Job drawing, mm, ordinate dimensions from the low corner. One solid piece. A direction names the side the tool comes from. Coordinates: 2 decimals unless noted, no trailing zeros. Order: outer loops, then holes, each group sorted by start corner. A loop starts at its lowest first (then second) coordinate and runs counter-clockwise, first axis right, second up. Notation, with made-up numbers: M -16.5,-27 L -12.5,-27 A5 cw -12.5,-18 Z; hole C -37.5,62 d5. An arc over 180 degrees is marked long. Write item = value, one per line.
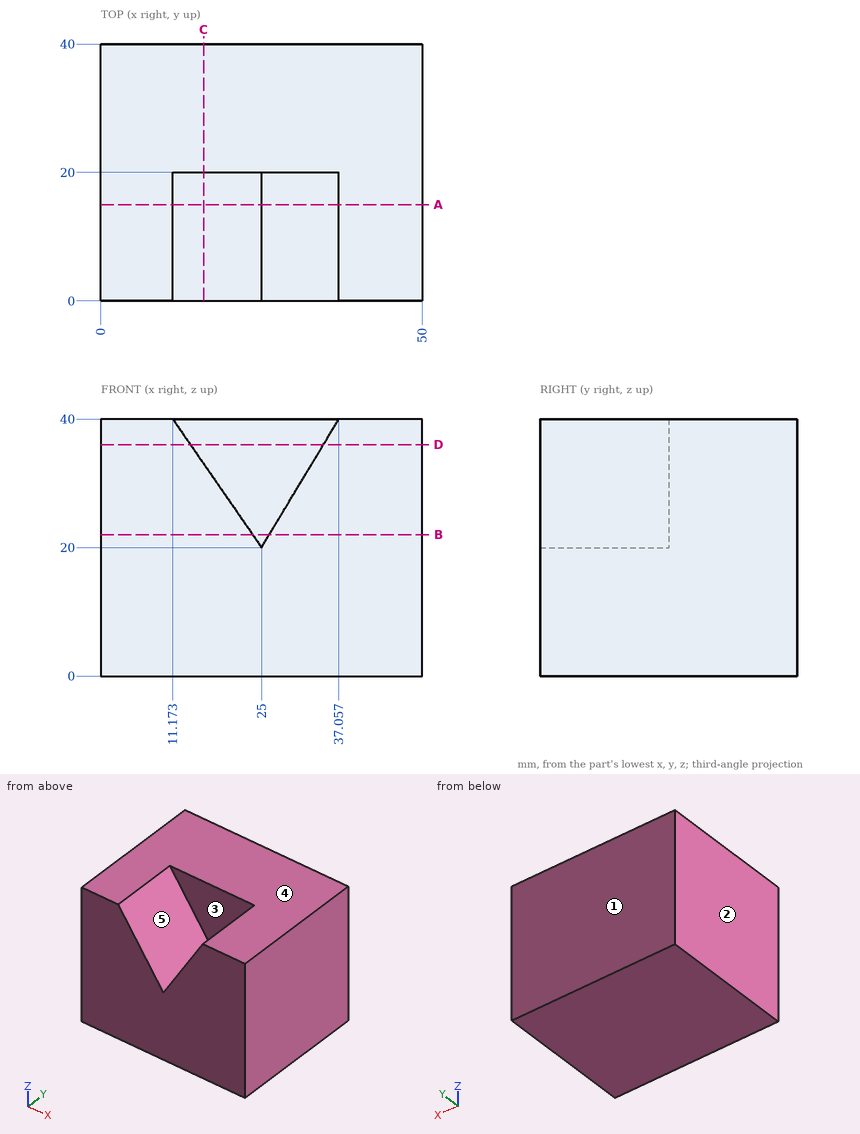
(1) Wall check: line 1 (Y direction, x = 27, z = 38.5); line 2 (X direction, y = 4, z = 26); line 3 (Z direction, x = 15, y = 13.5) (1 decimal). Give the ranges that are in metal, low to high. Write a range as from..to.
Evaluation:
line_1 = 20..40
line_2 = 0..20.85, 28.62..50
line_3 = 0..34.5
(2) Slice it at D-D, the plane z = 36. Write the cut outline in (x, y).
Evaluation:
outline = M 0,0 L 13.94,0 L 13.94,20 L 34.65,20 L 34.65,0 L 50,0 L 50,40 L 0,40 Z
(3) Tool access for the marked faces 4 and 5: list every direction of +Z, -Z, +X, -X, +Y, -Y with a clear straight run to the whole face (end or side of a thin tool).
Evaluation:
face_4 = +Z, +X, -X, +Y, -Y
face_5 = +Z, -Y
(4) Slice it at A-A, the plane y = 15. Write the cut outline in (x, z), then the cut area to 3 significant figures.
Evaluation:
outline = M 0,0 L 50,0 L 50,40 L 37.06,40 L 25,20 L 11.17,40 L 0,40 Z
area = 1,740 mm²
(5) Slice it at C-C, the plane x = 16. Write the cut outline in (y, z), then the cut area to 3 significant figures.
Evaluation:
outline = M 0,0 L 40,0 L 40,40 L 20,40 L 20,33.02 L 0,33.02 Z
area = 1,460 mm²
(6) Pull direction X, two halves, no side cores. Call the marked faces 1, 2 and 3: +X half, -X half, draft (parallel to the pull), parting line (faces both ways), or undercut.
Evaluation:
face_1 = draft
face_2 = -X half
face_3 = undercut
(7) Slice it at B-B, the plane z = 22. Write the cut outline in (x, y) (1 decimal), then the cut area to 3 significant figures.
Evaluation:
outline = M 0,0 L 23.6,0 L 23.6,20 L 26.2,20 L 26.2,0 L 50,0 L 50,40 L 0,40 Z
area = 1,950 mm²
(8) Pin check, flat tips, straight feed: pin 1 Ø1.5 at (x, y) = (31, 17.5) entering from +Z (1 decimal); pin 2 Ø10 at (x, z) = (25.5, 31) entering from -Y. Stop position of each tip, or through.
Evaluation:
pin_1 = 31.2
pin_2 = 20
